Geometry check sheet. Reference: the model listing, model coordinates, mm. Face numbers are marked on the shaded views. A direction names the side the tool comes from. Coordinates: 2 decimals unless noted, no trailing zeros. Write each loop counter-clockwise with the first axis right and the second up, starting at its lowest first coordinate (ties: lowest second). Pieces come first, ordered by that corner, then holes.
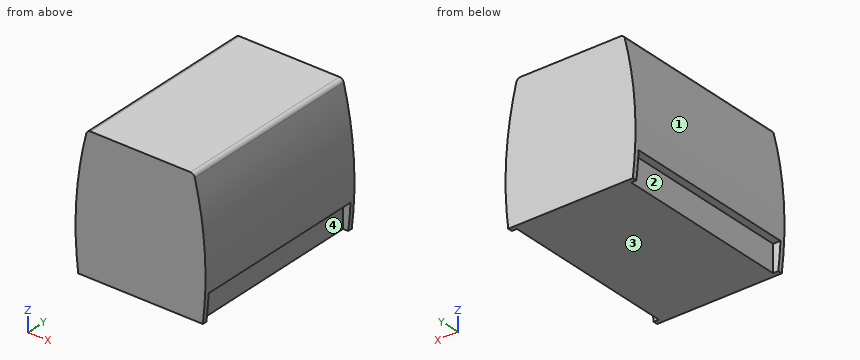
from build123d import *

# Parameters (mm, degrees)
F1_DEPTH = 1050
F2_W     = 200
F2_H     = 300
F3_DEPTH = 1000
F4_R     = 50


# Not quite as in the source:
# - a pattern or mirror of a feature is missing from the dataset's text; its kind, count and spacing are read off the source's solid


with BuildPart() as f1:
    # F0 (on Front) → F1 (new body, symmetric)
    with BuildSketch(Plane.XZ):
        with BuildLine():
            ThreePointArc((-600, 1500), (-721.1019148035, 754.7401276536), (-700, 0))
            Line((-700, 0), (700, 0))
            ThreePointArc((700, 0), (721.1019148035, 754.7401276536), (600, 1500))
            Line((600, 1500), (-600, 1500))
        make_face()
    extrude(amount=F1_DEPTH, both=True)

    # F2 (on Front) → F3 (cut, symmetric)
    with BuildSketch(Plane.XZ):
        with Locations((-742.0543789864, 150)):
            Rectangle(F2_W, F2_H)
    f3 = extrude(amount=F3_DEPTH, both=True, mode=Mode.SUBTRACT)

    # F3_copies: F3 across plane
    add(f3.mirror(Plane(origin=(0, 0, 0), x_dir=(0, 0, 1), z_dir=(1, 0, 0))), mode=Mode.SUBTRACT)

    # F4
    f4_edges = [f1.edges().sort_by_distance(p)[0] for p in [
        (600, 0, 1500),
        (-600, 0, 1500),
    ]]
    fillet(f4_edges, radius=F4_R)


solid = f1.part
1. Sectioned sample at A-A, the plane y = -876. Record the boundary of the cut face in (x, z).
Computed values:
outline: (-725.51, 300) - (-642.05, 300) - (-642.05, 0) - (642.05, 0) - (642.05, 300) - (725.51, 300) arc R4000 ccw to (609.69, 1462.17) arc R50 ccw to (561.19, 1500) - (-561.19, 1500) arc R50 ccw to (-609.69, 1462.17) arc R4000 ccw to start
2. Thickness scan on line 1 along X through (y, z) = (254, 143); line 2 along X through (y, z) = (15.5, 371.5); line 3 along Z through (x, y) = (585, -6.5). Record the ranges inside material, lowest first.
Computed values:
line 1: x = -642.05 to 642.05
line 2: x = -728.24 to 728.24
line 3: z = 0 to 1493.97
3. Sectioned sample at C-C, the plane z = 1100.5. Record the boundary of the cut face in (x, y).
Computed values:
outline: (-682.89, -1050) - (682.89, -1050) - (682.89, 1050) - (-682.89, 1050) - close
4. Sectioned sample at D-D, the plane z = 1341.5. Record the boundary of the cut face in (x, y), and give its area (3 significant figures).
Computed values:
outline: (-637.99, -1050) - (637.99, -1050) - (637.99, 1050) - (-637.99, 1050) - close
area: 2,680,000 mm2
5. Gauge pin test, flat end, axial feed: pin 1 Ø25 at (x, y) = (675, 457) entering from -Z. Record the tip position at first contact, or that the pin passes through.
Computed values:
pin 1: stops at z = 300
6. Access from +Z, -Z, +X, -X, +Y, -Y to the whole of each face (thin tool, end or side, straight path). Record for the marked faces 1, 2, 3 and 4.
Computed values:
face 1: -X, +Y, -Y
face 2: -Z, -X
face 3: -Z, +X, -X, +Y, -Y
face 4: -Z, +X
7. Sectioned sample at B-B, the plane z = 130.5. Record the boundary of the cut face in (x, y), and give its area (3 significant figures).
Computed values:
outline: (-713.89, -1050) - (713.89, -1050) - (713.89, -1000) - (642.05, -1000) - (642.05, 1000) - (713.89, 1000) - (713.89, 1050) - (-713.89, 1050) - (-713.89, 1000) - (-642.05, 1000) - (-642.05, -1000) - (-713.89, -1000) - close
area: 2,710,000 mm2
